Autodesk Inventor part; units mm, degrees
ref_plane "YZ Plane" through (0, 0, 0) normal (1, 0, 0) x (0, 1, 0)
ref_plane "XZ Plane" through (0, 0, 0) normal (0, 1, 0) x (-1, 0, 0)
ref_plane "XY Plane" through (0, 0, 0) normal (0, 0, 1) x (1, 0, 0)
sketch "Sketch1" plane through (0, 0, 0) normal (0, 0, 1) x (1, 0, 0)
  line L0 (0, 0) -> (36, 0)
  line L1 (36, 0) -> (36, 12)
  line L2 (36, 12) -> (24, 12)
  line L3 (24, 12) -> (24, 22)
  line L4 (24, 22) -> (12, 22)
  line L5 (12, 22) -> (12, 12)
  line L6 (12, 12) -> (0, 12)
  line L7 (0, 12) -> (0, 0)
  dimension "d0" = 36
  dimension "d1" = 12
  dimension "d2" = 12
  dimension "d3" = 10
  dimension "d4" = 12
extrude "Extrusion1" add sketch "Sketch1" along normal blind 108
sketch "Sketch2" plane through (0, 0, 0) normal (0, -1, 0) x (1, 0, 0)
  circle A0 centre (18, 4.5) radius 1.725
  line L0 (0, 0) -> (36, 0)
  line L1 (36, 0) -> (36, 108)
  circle A1 centre (18, 103.5) radius 1.725
  line L2 (0, 108) -> (36, 108)
  dimension "d7" = 3.45
  dimension "d8" = 4.5
  dimension "d9" = 18
  dimension "d10" = 3.45
  dimension "d11" = 18
  dimension "d12" = 4.5
extrude "Extrusion2" cut sketch "Sketch2" against normal blind 20
sketch "Sketch3" plane through (12, 22, 0) normal (0, 1, 0) x (1, 0, 0)
  circle A0 centre (6, -4.5) radius 1.725
  circle A1 centre (6, -4.5) radius 3
  circle A2 centre (6, -103.5) radius 1.725
  circle A3 centre (6, -103.5) radius 3
  point P0 (-12, 0)
  dimension "d15" = 6
  dimension "d16" = 6
extrude "Extrusion3" cut sketch "Sketch3" against normal blind 2 contours A0 | A1 | A2 | A3
sketch "Sketch4" plane through (36, 0, 0) normal (1, 0, 0) x (0, 0, -1)
  line L0 (-108, 0) -> (-107.85, 0)
  line L1 (0, 0) -> (-108, 0)
  line L2 (-107.85, 0) -> (-107.85, 12)
  line L3 (0, 12) -> (-108, 12)
  line L4 (-108, 0) -> (-108, 12)
  line L5 (-108, 12) -> (-108, 0)
  line L6 (-108, 22) -> (-107.85, 22)
  line L7 (-107.85, 12) -> (-108, 12)
  line L8 (0, 0) -> (-0.15, 0)
  line L9 (-0.15, 0) -> (-0.15, 12)
  line L10 (-0.15, 12) -> (0, 12)
  line L11 (0, 12) -> (0, 0)
  line L12 (0, 22) -> (-0.15, 22)
  line L13 (-0.15, 12) -> (0, 12)
  dimension "d19" = 0.15
  dimension "d20" = 12
  dimension "d21" = 0.15
  dimension "d22" = 0.15
extrude "Extrusion4" cut sketch "Sketch4" against normal through all contours L4 L3 L2 L0 | L9 L3 L11 L1
sketch "Sketch5" plane through (24, 22, 108) normal (1, 0, 0) x (0, 0, -1)
  line L0 (108, -10) -> (108, 0)
  line L1 (108, 0) -> (0, 0)
  line L2 (108, -10) -> (107.85, -10)
  line L3 (107.85, -10) -> (107.85, 0)
  line L4 (107.85, 0) -> (108, 0)
  line L5 (108, 0) -> (108, -10)
  line L6 (0.15, -10) -> (0, -10)
  line L7 (0, -10) -> (0, 0)
  line L8 (0.15, -10) -> (0, -10)
  line L9 (0, -10) -> (0, 0)
  line L10 (0, 0) -> (0.15, 0)
  line L11 (0.15, 0) -> (0.15, -10)
  point P0 (108, -22)
  dimension "d25" = 0.15
extrude "Extrusion5" cut sketch "Sketch5" against normal through all
sketch "Sketch6" plane through (12, 22, 0.15) normal (0, 1, 0) x (1, 0, 0)
  point P0 (0, -107.7)
sketch "Sketch7" plane through (0, 0, 107.85) normal (0, -1, 0) x (1, 0, 0)
  line L0 (0, -107.7) -> (36, -107.7)
  line L1 (11.85, -107.7) -> (24.15, -107.7)
  line L2 (24.15, -107.7) -> (24.15, -98.55)
  line L3 (24.15, -98.55) -> (11.85, -98.55)
  line L4 (11.85, -98.55) -> (11.85, -107.7)
  line L5 (0, 0) -> (12, 0)
  line L6 (11.85, 0) -> (24.15, 0)
  line L7 (24.15, 0) -> (24.15, -9.15)
  line L8 (24.15, -9.15) -> (11.85, -9.15)
  line L9 (11.85, -9.15) -> (11.85, 0)
  line L10 (36, -107.7) -> (36, 0)
  point P0 (0, -107.85)
  dimension "d30" = 11.85
  dimension "d31" = 11.85
  dimension "d32" = 9.15
  dimension "d33" = 11.85
  dimension "d34" = 11.85
  dimension "d35" = 9.15
extrude "Extrusion6" cut sketch "Sketch7" against normal blind 6
sketch "Sketch8" plane through (36, 0, 0.15) normal (0, -1, 0) x (1, 0, 0)
  line L0 (-21, 95.7) -> (-15, 95.7)
  line L1 (-15, 95.7) -> (-15, 12)
  line L2 (-15, 12) -> (-21, 12)
  line L3 (-21, 12) -> (-21, 95.7)
  line L4 (-11.85, 0) -> (-24.15, 0)
  line L5 (0, 107.7) -> (-11.85, 107.7)
  line L6 (-24, 0) -> (-24, 107.7)
  line L7 (-12, 0) -> (-12, 107.7)
  point P0 (-36, -0.15)
  dimension "d38" = 12
  dimension "d39" = 12
  dimension "d40" = 3
  dimension "d41" = 3
extrude "Extrusion7" cut sketch "Sketch8" against normal through all
sketch "Sketch9" plane through (24, 12, 107.85) normal (0, 1, 0) x (1, 0, 0)
  line L0 (9, 3) -> (0, 3)
  line L1 (0, 3) -> (0, 104.7)
  line L2 (0, 104.7) -> (9, 104.7)
  line L3 (9, 104.7) -> (9, 3)
  line L4 (-12, 3) -> (-21, 3)
  line L5 (-21, 3) -> (-21, 104.7)
  line L6 (-21, 104.7) -> (-12, 104.7)
  line L7 (-12, 104.7) -> (-12, 3)
  line L8 (12, 0) -> (0.15, 0)
  line L9 (12, 107.7) -> (0, 107.7)
  line L10 (12, 107.7) -> (12, 0)
  line L11 (-24, 107.7) -> (-24, 0)
  line L12 (-12, 107.7) -> (-24, 107.7)
  line L13 (-24, 0) -> (-12, 0)
  line L14 (-12, 107.7) -> (-12, 0)
  line L15 (0, 107.7) -> (0, 0)
  point P0 (-24, 107.85)
  dimension "d44" = 3
  dimension "d45" = 3
  dimension "d46" = 3
  dimension "d47" = 3
  dimension "d48" = 3
  dimension "d49" = 3
  dimension "d50" = 0
  dimension "d51" = 0
extrude "Extrusion8" cut sketch "Sketch9" against normal through all contours L0 L1 L2 L3 | L4 L5 L6 L7
sketch "Sketch10" plane through (12, 0, 98.7) normal (0, -1, 0) x (1, 0, 0)
  line L0 (3, -86.55) -> (3, -2.85)
  line L1 (9, -2.85) -> (9, -86.55)
  line L2 (3, -2.85) -> (9, -2.85)
  line L3 (9, -2.85) -> (9, -86.55)
  line L4 (9, -86.55) -> (3, -86.55)
  line L5 (3, -86.55) -> (3, -2.85)
  line L6 (0, 0) -> (0, -89.4)
  line L7 (0, 0) -> (12, 0)
  line L8 (12, 0) -> (12, -89.4)
  line L9 (12, -89.4) -> (0, -89.4)
  line L10 (0, -89.4) -> (0, 0)
  line L11 (12, -89.4) -> (0, -89.4)
  line L12 (0, -89.4) -> (0, 0)
  line L13 (0, 0) -> (12, 0)
  line L14 (12, 0) -> (12, -89.4)
  point P0 (-12, -98.7)
sketch "Sketch11" plane through (24, 12, 0.15) normal (1, 0, 0) x (0, 0, -1)
  line L0 (-107.7, 0) -> (-107.7, 10)
  line L1 (0, 0) -> (-107.7, 0)
  line L2 (-107.7, 10) -> (0, 10)
  line L3 (0, 10) -> (0, 0)
  line L4 (0, 0) -> (-107.7, 0)
  line L5 (-107.7, 0) -> (-107.7, 10)
  point P0 (0.15, -12)
extrude "Extrusion9" cut sketch "Sketch11" against normal through all
sketch "Sketch12" plane through (0, 12, 107.85) normal (0, 1, 0) x (1, 0, 0)
  circle A0 centre (18, 103.35) radius 1.725
  circle A1 centre (18, 103.35) radius 3
  circle A2 centre (18, 4.35) radius 1.725
  circle A3 centre (18, 4.35) radius 3
  point P0 (0, 107.85)
  dimension "d56" = 6
  dimension "d57" = 6
extrude "Extrusion10" cut sketch "Sketch12" against normal blind 2
sketch "Sketch13" plane through (0, 12, 107.85) normal (0, 1, 0) x (1, 0, 0)
  line L0 (36, 107.7) -> (0, 107.7)
  line L1 (36, 0) -> (0, 0)
  line L2 (36, 107.7) -> (24, 107.7)
  line L3 (24, 107.7) -> (24, 0)
  line L4 (24, 0) -> (36, 0)
  line L5 (36, 0) -> (36, 107.7)
  point P0 (0, 107.85)
  dimension "d60" = 12
extrude "Extrusion11" cut sketch "Sketch13" against normal through all
properties part number "topCutCenterBeam"
Design review of the part built by this model. Coordinates are the model's own, in mm. A direction names the side the tool comes from. Coordinates: 2 decimals unless noted, no trailing zeros. Order: outer loops, then holes, each group sorted by start corner. A loop starts at its lowest first (then second) coordinate and runs counter-clockwise, first axis right, second up.
1) Wall thickness on line 1 along Z through (x, y) = (18, 11.25); line 2 along Z through (x, y) = (18, 7.05) (3 decimals); line 3 along X through (y, z) = (8.65, 4.5) (3 decimals): over which ranges is each line inside the solid? List them lowest first.
2) Take a section at C-C, the plane x = 18. Give the boundary of the cut face in (y, z) (3 decimals), and give its area (3 significant figures).
3) Mouldability with a two-part tool opening along X and no side actions: class faces 5 (the flat face through (18, 3, 98.7)), 6 (the flat face through (24, 6, 53)), 7 (the flat face through (18, 6, 95.85)) as +X half, -X half, draft (parallel to the pull), parting line (faces both ways), or undercut.
4) Take a section at A-A, the plane z = 4.5. Give the boundary of the cut face in (x, y) (3 decimals).
5) Take a section at D-D, the plane y = 8.5. Give the boundary of the cut face in (x, z) (3 decimals), and give its area (3 significant figures).
6) Take a section at B-B, the plane x = 4.25. Give the boundary of the cut face in (y, z).
7) For faces 1 (the flat face through (20, 10, 4)), 2 (the flat face through (8, 6, 104.85)), 3 (the flat face through (11.85, 3, 106)), 4 (the flat face through (16, 6, 6)), list the 3-axis set-ups (+Z, -Z, +X, -X, +Y, -Y) from which the entire face can be reached by the end or side of a thin tool; tool diameter is ignored.
8) Clearance check with flat-ended pins moving along their axes: pin 1 (5 mm diameter, centred on x = 18, z = 103.5, fed in from -Y); pin 2 (3 mm diameter, centred on x = 17.5, z = 44, fed in from -Y); pin 3 (4 mm diameter, centred on x = 18, z = 4.5, fed in from +Y); pin 4 (3.5 mm diameter, centred on y = 4, z = 1.5, fed in from +X). State where each tip first meets the part, or that it passes through.
Returned:
1. line 1: z = 0.15 to 1.5, 7.5 to 12.15, 95.85 to 100.5, 106.5 to 107.85
1. line 2: z = 0.15 to 2.775, 6.225 to 12.15, 95.85 to 101.775, 105.225 to 107.85
1. line 3: x = 0 to 3, 12 to 16.275, 19.725 to 24
2. outline: (0, 9.3) - (6, 9.3) - (6, 6.225) - (10, 6.225) - (10, 7.5) - (12, 7.5) - (12, 12.15) - (0, 12.15) - close; (0, 95.85) - (12, 95.85) - (12, 100.5) - (10, 100.5) - (10, 101.775) - (6, 101.775) - (6, 98.7) - (0, 98.7) - close; (6, 0.15) - (12, 0.15) - (12, 1.5) - (10, 1.5) - (10, 2.775) - (6, 2.775) - close; (6, 105.225) - (10, 105.225) - (10, 106.5) - (12, 106.5) - (12, 107.85) - (6, 107.85) - close
2. area: 127 mm2
3. face 5: draft
3. face 6: +X half
3. face 7: undercut
4. outline: (0, 0) - (3, 0) - (3, 12) - (0, 12) - close; (12, 6) - (16.275, 6) - (16.275, 10) - (15, 10) - (15, 12) - (12, 12) - close; (19.725, 6) - (24, 6) - (24, 12) - (21, 12) - (21, 10) - (19.725, 10) - close
5. outline: (0, 0.15) - (24, 0.15) - (24, 107.85) - (0, 107.85) - close; hole (3, 3.15) - (12, 3.15) - (12, 104.85) - (3, 104.85) - close; hole (15, 12.15) - (21, 12.15) - (21, 95.85) - (15, 95.85) - close; hole circle Ø3.45 at (18, 4.5); hole circle Ø3.45 at (18, 103.5)
5. area: 1,150 mm2
6. outline: (0, 0.15) - (12, 0.15) - (12, 3.15) - (0, 3.15) - close; (0, 104.85) - (12, 104.85) - (12, 107.85) - (0, 107.85) - close
7. face 1: +Y
7. face 2: +Y, -Y
7. face 3: +Z, -Z, +X, -Y
7. face 4: -Z, +X, -Y
8. pin 1: stops at y = 6
8. pin 2: passes through
8. pin 3: stops at y = 10
8. pin 4: stops at x = 11.85
